```python
from build123d import *

# Parameters (mm, degrees)
F0_R     = 11.90625
F1_DEPTH = 1.5875
F2_R     = 10.31875
F3_DEPTH = 4.7625
F4_R     = 4.7625
F5_DEPTH = 3.175


# Not quite as in the source:
# - a length typed as a fraction of an inch, garbled in the dataset ("3 / 203.2 mm" for 3/8 in), is restored


with BuildPart() as f1:
    # F0 (on Front) → F1 (new body)
    with BuildSketch(Plane.XZ):
        Circle(F0_R)
    extrude(amount=F1_DEPTH)

    # F2 (on face) → F3 (join)
    with BuildSketch(Plane.XZ.offset(1.5875)):
        Circle(F2_R)
    extrude(amount=F3_DEPTH)

    # F4 (on face) → F5 (join)
    with BuildSketch(Plane.XZ.offset(6.35)):
        with Locations((-3.571875, 0)):
            Circle(F4_R)
    extrude(amount=F5_DEPTH)


solid = f1.part
```
Input: part model. Units: mm. Frame: model coordinates. A direction names the side the tool comes from. Give positions to 0.01 mm unless a question says otherwise; leave off trailing zeros. Loops run counter-clockwise (first coordinate to the right, second up) from the corner with the lowest first, then second, coordinate; pieces in that order, holes last. Notation, with made-up numbers: (-17, -35.75) -> (-6, -35.75) arc R13 ccw to (-6, -14.75) -> close; hole circle Ø5 at (9, 85). An arc over 180 degrees is marked (long way). Use a Markdown table: item, result.
Q1. Section query A-A, the plane z = -10. Return the cut outline in (x, y), plus the area to 3 significant figures.
Entries:
| item | result |
|---|---|
| outline | (-6.46, -1.59) -> (-2.54, -1.59) -> (-2.54, -6.35) -> (2.54, -6.35) -> (2.54, -1.59) -> (6.46, -1.59) -> (6.46, 0) -> (-6.46, 0) -> close |
| area | 44.8 mm² |
Q2. First-contact query: P1, Ø1.5, axis at x = 2.5, y = -1.5, coming from the -Z side; P2, Ø12, axis at x = 4, z = -8, coming from the -Y side; P3, Ø1.5, axis at x = -9, y = -2.5, coming from the +Z side. Flat tips, straight axial feed; report the tip coordinate or a pass-through.
Entries:
| item | result |
|---|---|
| P1 | stops at z = -11.78 |
| P2 | stops at y = -6.35 |
| P3 | stops at z = 6.2 |
Q3. Access query for faces 3 (the cylindrical face through (-9.45, -0.78, -7.24)), 4 (the cylindrical face through (-2.237, -3.935, -10.073)). Directions: +Z, -Z, +X, -X, +Y, -Y. A direction counts if a zero-diameter tool reaches every point of the face in a straight line with its end or side. Return the directions, or none.
Entries:
| item | result |
|---|---|
| face 3 | +Y, -Y |
| face 4 | -Y |
Q4. Ray query, probe 1 along Y at (x, z) = (-2, -4.75); probe 2 along Y at (x, z) = (-3.75, 10.25); probe 3 along X at (y, z) = (-7.5, -4.25). Return the intervals inside material, ascending. Write a range as from..to.
Entries:
| item | result |
|---|---|
| probe 1 | y = -6.35..0 |
| probe 2 | y = -1.59..0 |
| probe 3 | x = -5.72..-1.42 |
Q5. Pull-direction query (X, two-part tool) for faces 1 (the cylindrical face through (-7.35, -7.92, -2.9)), 2 (the flat face through (0, 0, 0)); classes: pulls with the +X half, pulls with the -X half, needs draft (parallel to the pull), parting line crosses it, or undercut.
Entries:
| item | result |
|---|---|
| face 1 | parting line crosses it |
| face 2 | needs draft |
Q6. Section query B-B, the plane y = -8. Return the cut outline in (x, z) (1 decimal).
Entries:
| item | result |
|---|---|
| outline | circle Ø9.5 at (-3.6, 0) |
